```python
from build123d import *

# Parameters (mm, degrees)
SKETCH1_R               = 7.9375
SKETCH1_R_2             = 11.1125
BOSS_EXTRUDE1_DEPTH     = 12.7
F_8_CLEARANCE_HOLE1_D   = 4.4958
SKETCH5_R               = 18.415
CUT_EXTRUDE1_DEPTH      = 13.7
SKETCH7_R               = 9.525
CUT_EXTRUDE2_DEPTH      = 13.7
CUT_EXTRUDE3_DEPTH      = 13.7
BOSS_EXTRUDE2_DEPTH     = 12.7
CUT_EXTRUDE4_DEPTH      = 13.7
SKETCH11_W              = 12.7
SKETCH11_H              = 178.054
CUT_EXTRUDE5_DEPTH      = 3.175
BOSS_EXTRUDE3_DEPTH     = 19.05
CUT_EXTRUDE6_DEPTH      = 20.05
F_3_8_CLEARANCE_HOLE1_D = 10.0838
CUT_EXTRUDE7_DEPTH      = 20.05
BOSS_EXTRUDE4_DEPTH     = 19.05
FILLET1_R               = 19.05
FILLET3_R               = 1.5875


with BuildPart() as part:
    # Sketch1 → Boss-Extrude1 (new body)
    with BuildSketch(Plane(origin=(0, 0, 0), x_dir=(0, 0, -1), z_dir=(1, 0, 0))):
        with BuildLine():
            Line((93.345, 0), (55.245, 50.8))
            Line((55.245, 50.8), (-160.655, 50.8))
            ThreePointArc((-160.655, 50.8), (-211.455, 0), (-160.655, -50.8))
            Line((-160.655, -50.8), (55.245, -50.8))
            Line((55.245, -50.8), (93.345, 0))
        make_face()
        with Locations((-88.9, 0)):
            Circle(SKETCH1_R, mode=Mode.SUBTRACT)
        with Locations((-38.1, 0)):
            Circle(SKETCH1_R, mode=Mode.SUBTRACT)
        with Locations((-160.655, 0)):
            Circle(SKETCH1_R_2, mode=Mode.SUBTRACT)
        Circle(SKETCH1_R, mode=Mode.SUBTRACT)
    extrude(amount=BOSS_EXTRUDE1_DEPTH)

    # #8 Clearance Hole1 (through all)
    with Locations(Plane.ZY):
        with Locations((-17.691104559, 17.691104559), (17.691104559, 17.691104559), (17.691104559, -17.691104559), (-17.691104559, -17.691104559)):
            Hole(F_8_CLEARANCE_HOLE1_D / 2)

    # Sketch5 → Cut-Extrude1 (cut, through all)
    with BuildSketch(Plane.ZY):
        Circle(SKETCH5_R)
    extrude(amount=-CUT_EXTRUDE1_DEPTH, mode=Mode.SUBTRACT)

    # Sketch7 → Cut-Extrude2 (cut, through all)
    with BuildSketch(Plane.ZY):
        with Locations((-55.245, 0)):
            Circle(SKETCH7_R)
    extrude(amount=-CUT_EXTRUDE2_DEPTH, mode=Mode.SUBTRACT)

    # Sketch8 → Cut-Extrude3 (cut, through all)
    with BuildSketch(Plane(origin=(12.7, 0, 0), x_dir=(0, 0, -1), z_dir=(1, 0, 0))):
        Polygon((-160.655, 50.8), (-211.455, 25.4), (-211.455, -25.4), (-160.655, -50.8), (-233.239745749, -50.8), (-233.239745749, 50.8), align=None)
    extrude(amount=-CUT_EXTRUDE3_DEPTH, mode=Mode.SUBTRACT)

    # Sketch9 → Boss-Extrude2 (add)
    with BuildSketch(Plane(origin=(12.7, 0, 0), x_dir=(0, 0, -1), z_dir=(1, 0, 0))):
        Polygon((-160.655, 50.8), (-211.455, 25.4), (-211.455, 0), (-211.455, -25.4), (-160.655, -50.8), (-160.655, -40.64), (-202.749323348, 0), (-160.655, 40.64), align=None)
    extrude(amount=-BOSS_EXTRUDE2_DEPTH)

    # Sketch10 → Cut-Extrude4 (cut, through all)
    with BuildSketch(Plane.ZY):
        Polygon((-79.0575, -19.05), (-79.0575, 19.05), (-93.345, 0), align=None)
    extrude(amount=-CUT_EXTRUDE4_DEPTH, mode=Mode.SUBTRACT)

    # Sketch11 → Cut-Extrude5 (cut)
    with BuildSketch(Plane(origin=(0, 50.8, 0), x_dir=(1, 0, 0), z_dir=(0, 1, 0))):
        with Locations((6.35, -52.705)):
            Rectangle(SKETCH11_W, SKETCH11_H)
    cut_extrude5 = extrude(amount=-CUT_EXTRUDE5_DEPTH, mode=Mode.SUBTRACT)

    # Mirror1: Cut-Extrude5 across plane
    add(cut_extrude5.mirror(Plane.ZX), mode=Mode.SUBTRACT)

    # Sketch13 → Cut-Extrude6 (cut, through all)
    with BuildSketch(Plane(origin=(12.7, 0, 0), x_dir=(0, 0, -1), z_dir=(1, 0, 0))):
        Polygon((-161.254612663, -53.34), (-139.192, -53.34), (-139.192, -50.165), (33.782, -50.165), (33.782, -53.34), (56.515, -53.34), (81.5975, -19.896666667), (81.5975, 19.896666667), (56.515, 53.34), (33.782, 53.34), (33.782, 50.165), (-139.192, 50.165), (-139.192, 53.34), (-161.254612663, 53.34), (-213.995, 26.969806331), (-213.995, -26.969806331), align=None)
    extrude(amount=-CUT_EXTRUDE6_DEPTH, mode=Mode.SUBTRACT)


with BuildPart() as body_2:
    # Sketch12 → Boss-Extrude3 (new body)
    with BuildSketch(Plane(origin=(12.7, 0, 0), x_dir=(0, 0, -1), z_dir=(1, 0, 0))):
        with BuildLine():
            ThreePointArc((-211.89681554, -56.397839854), (-236.855, 0), (-211.89681554, 56.397839854))
            Line((-211.89681554, 56.397839854), (-243.205, 43.989212666))
            Line((-243.205, 43.989212666), (-243.205, -43.989212666))
            Line((-243.205, -43.989212666), (-211.89681554, -56.397839854))
        make_face()
        with BuildLine():
            Line((-217.805, 29.324515829), (-162.154031657, 57.15))
            Line((-162.154031657, 57.15), (-166.916531657, 66.675))
            Line((-166.916531657, 66.675), (-185.966531657, 66.675))
            Line((-185.966531657, 66.675), (-211.89681554, 56.397839854))
            ThreePointArc((-211.89681554, 56.397839854), (-236.855, 0), (-211.89681554, -56.397839854))
            Line((-211.89681554, -56.397839854), (-185.966531657, -66.675))
            Line((-185.966531657, -66.675), (-166.916531657, -66.675))
            Line((-166.916531657, -66.675), (-162.154031657, -57.15))
            Line((-162.154031657, -57.15), (-217.805, -29.324515829))
            Line((-217.805, -29.324515829), (-217.805, 29.324515829))
        make_face()
    extrude(amount=-BOSS_EXTRUDE3_DEPTH)

    # 3/8 Clearance Hole1 (through all)
    with Locations(Plane(origin=(12.7, 0, 0), x_dir=(0, 0, -1), z_dir=(1, 0, 0))):
        with Locations((-230.505, 0), (-230.505, 33.690140829), (-202.106936686, 47.889172486), (-230.505, -33.690140829), (-202.106936686, -47.889172486)):
            Hole(F_3_8_CLEARANCE_HOLE1_D / 2)

    # Sketch16 → Cut-Extrude7 (cut, through all)
    with BuildSketch(Plane(origin=(12.7, 0, 0), x_dir=(0, 0, -1), z_dir=(1, 0, 0))):
        with BuildLine():
            ThreePointArc((-190.589767426, 47.889172486), (-190.722432786, 46.146112328), (-191.117372542, 44.443208515))
            Line((-191.117372542, 44.443208515), (-162.86398324, 58.569903166))
            Line((-162.86398324, 58.569903166), (-166.916531657, 66.675))
            Line((-166.916531657, 66.675), (-185.966531657, 66.675))
            Line((-185.966531657, 66.675), (-206.35048523, 58.596062021))
            ThreePointArc((-206.35048523, 58.596062021), (-195.635015761, 57.415946719), (-190.589767426, 47.889172486))
        make_face()
        with BuildLine():
            Line((-162.86398324, 58.569903166), (-191.117372542, 44.443208515))
            ThreePointArc((-191.117372542, 44.443208515), (-191.551739911, 43.281243579), (-192.108559765, 42.172735946))
            Line((-192.108559765, 42.172735946), (-162.154031657, 57.15))
            Line((-162.154031657, 57.15), (-162.86398324, 58.569903166))
        make_face()
        with BuildLine():
            Line((-191.117372542, 44.443208515), (-205.943903995, 37.029942788))
            ThreePointArc((-205.943903995, 37.029942788), (-204.753711625, 36.680257722), (-203.532813606, 36.460609025))
            Line((-203.532813606, 36.460609025), (-192.108559765, 42.172735946))
            ThreePointArc((-192.108559765, 42.172735946), (-191.551739911, 43.281243579), (-191.117372542, 44.443208515))
        make_face()
        with BuildLine():
            Line((-219.3925, 30.305644786), (-219.3925, -30.305644786))
            Line((-219.3925, -30.305644786), (-205.943903995, -37.029942788))
            ThreePointArc((-205.943903995, -37.029942788), (-204.753711625, -36.680257722), (-203.532813606, -36.460609025))
            Line((-203.532813606, -36.460609025), (-217.805, -29.324515829))
            Line((-217.805, -29.324515829), (-217.805, 29.324515829))
            Line((-217.805, 29.324515829), (-203.532813606, 36.460609025))
            ThreePointArc((-203.532813606, 36.460609025), (-204.753711625, 36.680257722), (-205.943903995, 37.029942788))
            Line((-205.943903995, 37.029942788), (-219.3925, 30.305644786))
        make_face()
        with BuildLine():
            ThreePointArc((-203.532813606, -36.460609025), (-204.753711625, -36.680257722), (-205.943903995, -37.029942788))
            Line((-205.943903995, -37.029942788), (-191.117372542, -44.443208515))
            ThreePointArc((-191.117372542, -44.443208515), (-191.551739911, -43.281243579), (-192.108559765, -42.172735946))
            Line((-192.108559765, -42.172735946), (-203.532813606, -36.460609025))
        make_face()
        with BuildLine():
            ThreePointArc((-192.108559765, -42.172735946), (-191.551739911, -43.281243579), (-191.117372542, -44.443208515))
            Line((-191.117372542, -44.443208515), (-162.86398324, -58.569903166))
            Line((-162.86398324, -58.569903166), (-162.154031657, -57.15))
            Line((-162.154031657, -57.15), (-192.108559765, -42.172735946))
        make_face()
        with BuildLine():
            Line((-162.86398324, -58.569903166), (-191.117372542, -44.443208515))
            ThreePointArc((-191.117372542, -44.443208515), (-190.722432786, -46.146112328), (-190.589767426, -47.889172486))
            Line((-190.589767426, -47.889172486), (-190.589767426, -64.842635395))
            Line((-190.589767426, -64.842635395), (-185.966531657, -66.675))
            Line((-185.966531657, -66.675), (-166.916531657, -66.675))
            Line((-166.916531657, -66.675), (-162.86398324, -58.569903166))
        make_face()
    extrude(amount=-CUT_EXTRUDE7_DEPTH, mode=Mode.SUBTRACT)

    # Sketch17 → Boss-Extrude4 (add)
    with BuildSketch(Plane(origin=(12.7, 0, 0), x_dir=(0, 0, -1), z_dir=(1, 0, 0))):
        Polygon((-490.855, -72.564212666), (-210.072064852, -72.564212666), (-190.589767426, -64.842635395), (-243.205, -43.989212666), (-243.205, 43.989212666), (-255.905, 38.955718453), (-287.655, -34.464212666), (-586.105, -53.514212666), (-611.505, -72.564212666), (-497.205, -72.564212666), align=None)
    extrude(amount=-BOSS_EXTRUDE4_DEPTH)

    # Fillet1
    fillet1_edges = [body_2.edges().sort_by_distance(p)[0] for p in [
        (3.175, -72.564212666, 210.072064852),
        (3.175, -53.514212666, 586.105),
        (3.175, -34.464212666, 287.655),
        (3.175, 38.955718453, 255.905),
        (3.175, -64.842635395, 190.589767426),
    ]]
    fillet(fillet1_edges, radius=FILLET1_R)

    # Fillet3
    fillet3_edges = [body_2.edges().sort_by_distance(p)[0] for p in [
        (3.175, -72.564212666, 611.505),
    ]]
    fillet(fillet3_edges, radius=FILLET3_R)


solid = body_2.part
```
Here's how the part is built. I have some questions about the finished solid (model axes, mm). A direction names the side the tool comes from. Coordinates: 2 decimals unless noted, no trailing zeros. Order: outer loops, then holes, each group sorted by start corner. A loop starts at its lowest first (then second) coordinate and runs counter-clockwise, first axis right, second up.
1) Which directions (+Z, -Z, +X, -X, +Y, -Y) give clear straight access to the entire face, cutting with the end or side of a thin tool? Please do faces 4 (the face through (3.04, -54.32, 585.89)), 5 (the face through (3, 0, 219.392)).
2) Imagine slicing it at A-A on y = 0. List the corners of the cut face in (x, z) for me, and give its area (3 significant figures).
3) Imagine slicing it at C-C on z = 558. List the corners of the cut face in (x, y) for me.
4) Imagine slicing it at D-D on z = 352. List the corners of the cut face in (x, y) for me, and give its area (3 significant figures).
5) Imagine slicing it at B-B on x = 2.5. State how many separate pieces and enclosed holes the cut face has, and give its area (3 significant figures).
6) I need wall thicknesses on line 1 (Y direction, x = 1.5, z = 560); line 2 (Y direction, x = 8.25, z = 275.5); line 3 (Z direction, x = -5.5, y = 32). Which ranges of each line are inside material? Lowest first, please.
7) We'd pull the mould along Y, two halves only. Please class faces 1 (the face through (3.042, -62.737, 193.972)), 2 (the face through (3.042, -1.931, 235.162)), 3 (the face through (3.308, -44.054, 437.897)): +Y half, -Y half, draft (parallel to the pull), parting line (faces both ways), or undercut.
8) Will these pins go through, and if not, where does the flat tip stop? pin 1 (9.5 mm diameter, centred on x = 3.5, y = -9.5, fed in from -Z); pin 2 (8 mm diameter, centred on x = 2.5, z = 258, fed in from +Y).
Response values:
1. face 4: +Z, +X, -X, +Y
1. face 5: -Z, +X, -X
2. outline: (-6.35, 219.39) - (12.7, 219.39) - (12.7, 225.46) - (-6.35, 225.46) - close; (-6.35, 235.55) - (12.7, 235.55) - (12.7, 272.75) - (-6.35, 272.75) - close
2. area: 824 mm2
3. outline: (-6.35, -72.56) - (12.7, -72.56) - (12.7, -51.72) - (-6.35, -51.72) - close
4. outline: (-6.35, -72.56) - (12.7, -72.56) - (12.7, -38.57) - (-6.35, -38.57) - close
4. area: 648 mm2
5. separate pieces: 1
5. enclosed holes: 5
5. area: 16,500 mm2
6. line 1: y = -72.56 to -51.85
6. line 2: y = -72.56 to -6.36
6. line 3: z = 216 to 225.75, 235.26 to 258.91
7. face 1: -Y half
7. face 2: undercut
7. face 3: +Y half
8. pin 1: stops at z = 219.39
8. pin 2: stops at y = 38.57
